Could you check a few things on this model? Use its own coordinates, in mm. A direction names the side the tool comes from. Round coordinates to 2 decimals unless told otherwise and drop trailing zeros. Loops run counter-clockwise (first coordinate to the right, second up) from the corner with the lowest first, then second, coordinate; pieces in that order, holes last. Notation, with made-up numbers: M -20.75,-11.75 L 16.25,-11.75 A21 cw 16.25,24.25 Z; hole C 50,38 d11. An arc over 180 degrees is marked long. Answer in a Markdown table with one row per item.
```python
from build123d import *

# Parameters (mm, degrees)
SKETCH2_W           = 100
SKETCH2_H           = 60
BOSS_EXTRUDE1_DEPTH = 5
SKETCH4_W           = 28
SKETCH4_H           = 12.508
BOSS_EXTRUDE2_DEPTH = 2.5
SKETCH5_W           = 2.5
SKETCH5_H           = 12.508
BOSS_EXTRUDE3_DEPTH = 10


with BuildPart() as part:
    # Sketch2 → Boss-Extrude1 (new body)
    with BuildSketch(Plane(origin=(0, 0, 0), x_dir=(1, 0, 0), z_dir=(0, 1, 0))):
        Rectangle(SKETCH2_W, SKETCH2_H)
    extrude(amount=BOSS_EXTRUDE1_DEPTH)

    # Sketch4 → Boss-Extrude2 (add)
    with BuildSketch(Plane(origin=(0, 5, 0), x_dir=(1, 0, 0), z_dir=(0, 1, 0))):
        with Locations((-33.5, 0)):
            Rectangle(SKETCH4_W, SKETCH4_H)
        with Locations((33.5, 0)):
            Rectangle(SKETCH4_W, SKETCH4_H)
    extrude(amount=BOSS_EXTRUDE2_DEPTH)

    # Sketch5 → Boss-Extrude3 (add)
    with BuildSketch(Plane(origin=(0, 5, 0), x_dir=(1, 0, 0), z_dir=(0, 1, 0))):
        with Locations((-18.25, 0)):
            Rectangle(SKETCH5_W, SKETCH5_H)
        with Locations((18.25, 0)):
            Rectangle(SKETCH5_W, SKETCH5_H)
    extrude(amount=BOSS_EXTRUDE3_DEPTH)


solid = part.part
```
1) If we mould it in two halves opening along X, with no side actions, what happens to faces 1 (the face through (-19.5, 11, 0)), 2 (the face through (-17, 10, 0)), 3 (the face through (-18, 15, 0))? For each: released by +X, released by -X, zero draft, split by the parting line, or undercut.
Computed:
| item | result |
|---|---|
| face 1 | released by -X |
| face 2 | undercut |
| face 3 | zero draft |
2) I need wall thicknesses on line 1 (Y direction, x = -19, z = -23); line 2 (Y direction, x = 44.5, z = 4); line 3 (X direction, y = 10.75, z = 3). Which ranges of each line are inside material? Lowest first, please.
Computed:
| item | result |
|---|---|
| line 1 | y = 0 to 5 |
| line 2 | y = 0 to 7.5 |
| line 3 | x = -19.5 to -17, 17 to 19.5 |
3) I want a section at C-C, the plane z = -12. Please give me the cut outline in (x, y), plus the area to 3 significant figures.
Computed:
| item | result |
|---|---|
| outline | M -50,0 L 50,0 L 50,5 L -50,5 Z |
| area | 500 mm² |
4) Which directions (+Z, -Z, +X, -X, +Y, -Y) give clear straight access to the entire face, cutting with the end or side of a thin tool? Please do faces 4 (the face through (30, 7, -6.254)), 5 (the face through (-30, 7, 6.254)), 6 (the face through (19.5, 11, 0)).
Computed:
| item | result |
|---|---|
| face 4 | -Z, +X, -X, +Y |
| face 5 | +Z, +X, -X, +Y |
| face 6 | +Z, -Z, +X, +Y |
5) Will these pins go through, and if not, where does the flat tip stop? P1, Ø6, axis at y = 13, z = 3, coming from the +X side; P2, Ø5, axis at x = 32, y = 10.5, coming from the +Z side; P3, Ø6, axis at x = 26.5, y = 8.5, coming from the -Z side; P4, Ø6.5, axis at x = -35, z = 2, coming from the +Y side.
Computed:
| item | result |
|---|---|
| P1 | stops at x = 19.5 |
| P2 | passes through |
| P3 | stops at z = -6.25 |
| P4 | stops at y = 7.5 |
6) I want a section at B-B, the plane y = 10.75. Please give me the cut outline in (x, z).
Computed:
| item | result |
|---|---|
| outline | M -19.5,-6.25 L -17,-6.25 L -17,6.25 L -19.5,6.25 Z; M 17,-6.25 L 19.5,-6.25 L 19.5,6.25 L 17,6.25 Z |
7) I want a section at D-D, the plane x = -14. Please give me the cut outline in (y, z), plus the area to 3 significant figures.
Computed:
| item | result |
|---|---|
| outline | M 0,-30 L 5,-30 L 5,30 L 0,30 Z |
| area | 300 mm² |
8) I want a section at A-A, the plane x = -30.5. Please give me the cut outline in (y, z), plus the area to 3 significant figures.
Computed:
| item | result |
|---|---|
| outline | M 0,-30 L 5,-30 L 5,-6.25 L 7.5,-6.25 L 7.5,6.25 L 5,6.25 L 5,30 L 0,30 Z |
| area | 331 mm² |
